Can you work these out from the model? Positions are in its coordinate system, mm. A direction names the side the tool comes from. Give positions to 0.01 mm unless a question says otherwise; leave off trailing zeros. Write each loop counter-clockwise with the first axis right and the second up, starting at its lowest first coordinate (ties: lowest second). Pieces come first, ordered by that corner, then holes.
```python
from build123d import *

# Parameters (mm, degrees)
F1_DEPTH = 60
F3_DEPTH = 60.001
F5_DEPTH = 100.001
F6_R     = 5


with BuildPart() as f1:
    # F0 (on Top) → F1 (new body)
    with BuildSketch(Plane.XY):
        Polygon((0, 60), (0, 0), (20, 0), (20, 15), (55, 15), (55, 0), (70, 0), (70, 20), (100, 20), (100, 60), align=None)
    extrude(amount=F1_DEPTH)

    # F2 (on Front) → F3 (cut, through all)
    with BuildSketch(Plane.XZ):
        Polygon((15.358984, 40), (50, 60), (0, 60), (0, 40), align=None)
        Polygon((100, 60), (75, 60), (100, 35), align=None)
    extrude(amount=-F3_DEPTH, mode=Mode.SUBTRACT)

    # F4 (on Right) → F5 (cut, through all)
    with BuildSketch(Plane.YZ):
        Polygon((0, 5), (50, 60), (0, 60), align=None)
    extrude(amount=F5_DEPTH, mode=Mode.SUBTRACT)

    # F6
    f6_edges = [f1.edges().sort_by_distance(p)[0] for p in [
        (62.5, 50, 60),
        (87.5, 38.636364, 47.5),
    ]]
    fillet(f6_edges, radius=F6_R)


solid = f1.part
```
1) If we mould it in two halves opening along X, with no side actions, what happens to faces 5 (the face through (100, 40, 17)), 6 (the face through (49.3, 23.92, 31.31)), 7 (the face through (37, 15, 11))? For each: +X half, -X half, draft (parallel to the pull), parting line (faces both ways), or undercut.
Values follow:
face 5: +X half
face 6: draft
face 7: undercut
2) Suppose I cut it at A-A on y = 10.5. Write out the boundary of the cut face in (x, z), plus the area to 3 significant figures.
Values follow:
outline: (0, 0) - (20, 0) - (20, 16.55) - (0, 16.55) - close; (55, 0) - (70, 0) - (70, 16.55) - (55, 16.55) - close
area: 579 mm2
3) For faces 1 (the face through (8, 46, 40)), 2 (the face through (85, 20, 13)), 3 (the face through (20, 9, 8)), 4 (the face through (90, 48, 45)), which set-ups out of +Z, -Z, +X, -X, +Y, -Y let a thin tool reach every point of the face, with its end or its side?
Values follow:
face 1: +Z, -X, +Y, -Y
face 2: +Z, -Z, +X, -Y
face 3: +Z, -Z, -Y
face 4: +Z, +X, +Y, -Y
4) For pin 1 Ø1.5 at (x, y) = (78, 18.5) entering from +Z; pin 2 Ø10 at (x, y) = (88.5, 53.5) entering from -Z; pin 3 Ø1 at (x, z) = (73, 50) entering from -Y; pin 4 Ø7.5 at (y, z) = (7, 12.5) entering from +X, each with a flat end and sliding along its axis, tell me the tip position at first contact or that it passes through.
Values follow:
pin 1: passes through
pin 2: stops at z = 0
pin 3: stops at y = 40.45
pin 4: stops at x = 70
5) Please list where these lines run through material, in increasing order: L1, parallel to X at y = 6, z = 8.5; L2, parallel to Y at x = 47, z = 21.5; L3, parallel to Y at x = 72, z = 43.5.
Values follow:
L1: x = 0 to 20, 55 to 70
L2: y = 15 to 60
L3: y = 35 to 60
6) Suppose I cut it at D-D on x = 53. Write out the boundary of the cut face in (y, z), plus the area to 3 significant figures.
Values follow:
outline: (15, 0) - (60, 0) - (60, 60) - (52.21, 60) arc R5 ccw to (48.51, 58.36) - (15, 21.5) - close
area: 2,030 mm2
7) Suppose I cut it at B-B on y = 55. Write out the boundary of the cut face in (x, z), plus the area to 3 significant figures.
Values follow:
outline: (0, 0) - (100, 0) - (100, 35) - (75, 60) - (50, 60) - (15.36, 40) - (0, 40) - close
area: 5,030 mm2
8) Suppose I cut it at C-C on z = 17. Write out the boundary of the cut face in (x, y), plus the area to 3 significant figures.
Values follow:
outline: (0, 10.91) - (20, 10.91) - (20, 15) - (55, 15) - (55, 10.91) - (70, 10.91) - (70, 20) - (100, 20) - (100, 60) - (0, 60) - close
area: 4,490 mm2
